Check sheet for the drawn part. Datum: minimum x, y, z corner. Units: mm. Give positions to 0.01 mm unless a question says otherwise; leave off trailing zeros. Order: outer loops, then holes, each group sorted by start corner. A loop starts at its lowest first (then second) coordinate and runs counter-clockwise, first axis right, second up.
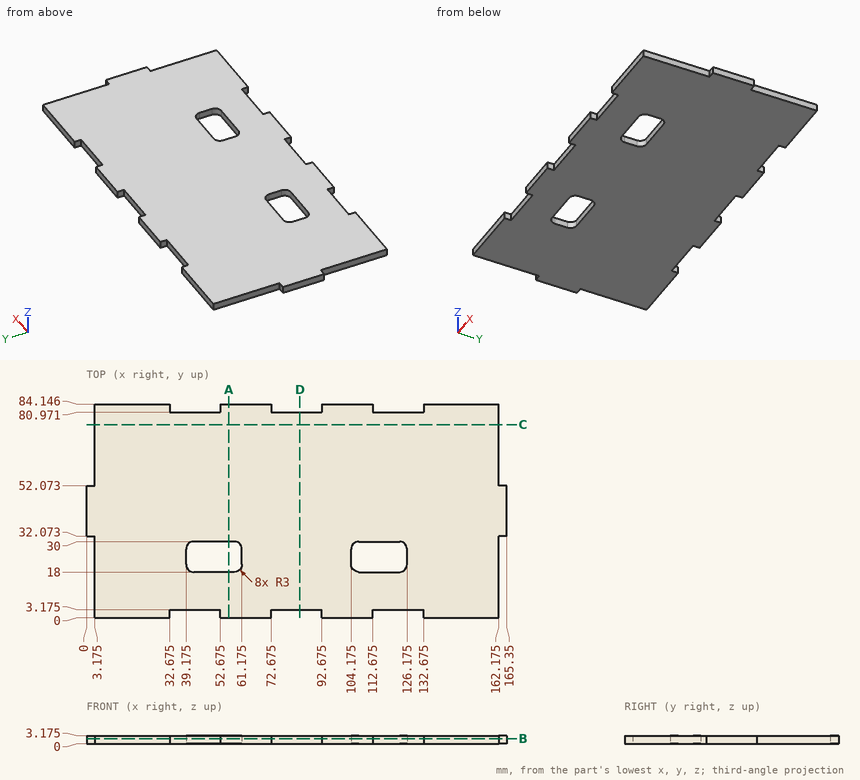
Item 1: Scan lines: L1, parallel to X at y = 23.5, z = 2.6 (3 decimals); L2, parallel to Y at x = 118.5, z = 1.7 (3 decimals); L3, parallel to X at y = 80.5, z = 1.75 (3 decimals). Record each from-to range of solid material in increasing order.
Reported:
L1: x = 3.175 to 39.175, 61.175 to 104.175, 126.175 to 162.175
L2: y = 3.175 to 18, 30 to 80.971
L3: x = 3.175 to 162.175
Item 2: Sectioned sample at B-B (z = 2.05). Give the number of separate pieces and of enclosed holes in the cut face, and give its area (3 significant figures).
Reported:
separate pieces: 1
enclosed holes: 2
area: 12,600 mm2
Item 3: Sectioned sample at D-D (x = 84). Enter the section's corners in (y, z) (3 decimals), and give its area (3 significant figures).
Reported:
outline: (3.175, 0) - (80.971, 0) - (80.971, 3.175) - (3.175, 3.175) - close
area: 247 mm2
Item 4: Sectioned sample at C-C (y = 76). Enter the section's corners in (x, z) (3 decimals).
Reported:
outline: (3.175, 0) - (162.175, 0) - (162.175, 3.175) - (3.175, 3.175) - close
Item 5: Sectioned sample at A-A (x = 56). Enter the section's corners in (y, z) (3 decimals), and give its area (3 significant figures).
Reported:
outline: (0, 0) - (18, 0) - (18, 3.175) - (0, 3.175) - close; (30, 0) - (84.146, 0) - (84.146, 3.175) - (30, 3.175) - close
area: 229 mm2
Item 6: Gauge pin test, flat ends, axial feed: pin 1 (1.6 mm diameter, centred on y = 24, z = 1.5, fed in from -X) (3 decimals); pin 2 (1.6 mm diameter, centred on x = 81.5, z = 1, fed in from +Y); pin 3 (1.6 mm diameter, centred on x = 163.5, z = 1.5, fed in from -Y). Record the tip position at first contact, or that the pin passes through.
Reported:
pin 1: stops at x = 3.175
pin 2: stops at y = 80.97
pin 3: stops at y = 32.07
